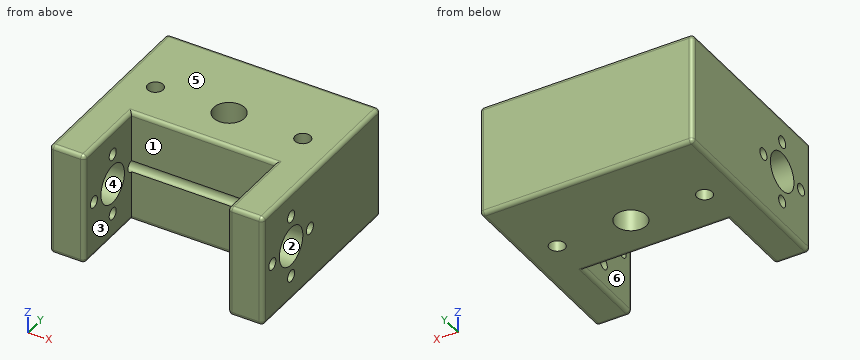
from build123d import *

# Parameters (mm, degrees)
BOSS_EXTRUDE1_DEPTH = 14.5
SKETCH2_R           = 5
SKETCH2_R_2         = 1.5
CUT_EXTRUDE1_DEPTH  = 63.130910182
SKETCH3_R           = 4
SKETCH3_R_2         = 2
CUT_EXTRUDE2_DEPTH  = 48.140746706
FILLET1_R           = 1


with BuildPart() as part:
    # Sketch1 → Boss-Extrude1 (new, symmetric)
    with BuildSketch(Plane.XY):
        Polygon((-27.5, -25), (-18.5, -25), (-18.5, -5), (18.5, -5), (18.5, -25), (27.5, -25), (27.5, 25), (-27.5, 25), align=None)
    extrude(amount=BOSS_EXTRUDE1_DEPTH, both=True)

    # Sketch2 → Cut-Extrude1 (cut, through all)
    with BuildSketch(Plane(origin=(27.5, 0, 0), x_dir=(0, 0, -1), z_dir=(1, 0, 0))):
        with Locations((0, -13)):
            Circle(SKETCH2_R)
        with Locations((0, -21)):
            Circle(SKETCH2_R_2)
        with Locations((-8, -13)):
            Circle(SKETCH2_R_2)
        with Locations((0, -5)):
            Circle(SKETCH2_R_2)
        with Locations((8, -13)):
            Circle(SKETCH2_R_2)
    extrude(amount=-CUT_EXTRUDE1_DEPTH, mode=Mode.SUBTRACT)

    # Sketch3 → Cut-Extrude2 (cut, through all)
    with BuildSketch(Plane.XY.offset(14.5)):
        with Locations((0, 6)):
            Circle(SKETCH3_R)
        with Locations((-19, 6)):
            Circle(SKETCH3_R_2)
        with Locations((19, 6)):
            Circle(SKETCH3_R_2)
    extrude(amount=-CUT_EXTRUDE2_DEPTH, mode=Mode.SUBTRACT)

    # Fillet1
    fillet1_edges = [part.edges().sort_by_distance(p)[0] for p in [
        (-18.5, -15, -14.5),
        (-23, -25, -14.5),
        (23, -25, 14.5),
        (-27.5, 0, -14.5),
        (0, 25, -14.5),
        (27.5, 0, -14.5),
        (23, -25, -14.5),
        (18.5, -15, -14.5),
        (27.5, 0, 14.5),
        (-18.5, -25, 0),
        (-27.5, -25, 0),
        (-27.5, 25, 0),
        (27.5, 25, 0),
        (27.5, -25, 0),
        (18.5, -25, 0),
        (0, 25, 14.5),
        (-27.5, 0, 14.5),
        (-23, -25, 14.5),
        (-18.5, -15, 14.5),
        (0, -5, 14.5),
        (18.5, -15, 14.5),
        (0, -5, -14.5),
    ]]
    fillet(fillet1_edges, radius=FILLET1_R)


solid = part.part
Verification items for the finished model (mm, model axes). Face numbers are marked on the shaded views. A direction names the side the tool comes from. Coordinates: 2 decimals unless noted, no trailing zeros. Order: outer loops, then holes, each group sorted by start corner. A loop starts at its lowest first (then second) coordinate and runs counter-clockwise, first axis right, second up.
Item 1: Release check for a two-part mould opening along Y. For the marked faces 1, 2, 3 and 4 record: +Y half, -Y half, draft (parallel to the pull), parting line (faces both ways), or undercut.
Filled in:
face 1: -Y half
face 2: undercut
face 3: draft
face 4: undercut
Item 2: Section check B-B, the plane x = 0. Enter the section's corners in (y, z), then the cut area to 3 significant figures.
Filled in:
outline: (-5, -13.5) arc R1 ccw to (-4, -14.5) - (2, -14.5) - (2, 14.5) - (-4, 14.5) arc R1 ccw to (-5, 13.5) - (-5, 1.5) arc R1.5 cw to (-5, -1.5) - close; (10, -14.5) - (24, -14.5) arc R1 ccw to (25, -13.5) - (25, 13.5) arc R1 ccw to (24, 14.5) - (10, 14.5) - close
area: 634 mm2
Item 3: Section check D-D, the plane y = 9. Enter the section's corners in (x, z).
Filled in:
outline: (-27.5, -13.5) arc R1 ccw to (-26.5, -14.5) - (-2.65, -14.5) - (-2.65, 14.5) - (-26.5, 14.5) arc R1 ccw to (-27.5, 13.5) - close; (2.65, -14.5) - (26.5, -14.5) arc R1 ccw to (27.5, -13.5) - (27.5, 13.5) arc R1 ccw to (26.5, 14.5) - (2.65, 14.5) - close
Item 4: Material ranges on L1, parallel to Y at x = -22.75, z = 0; L2, parallel to X at y = -10.5, z = 7.5; L3, parallel to X at y = 5, z = -10, recorded low to high.
Filled in:
L1: y = -25 to -22.5, -19.5 to -18, -8 to -6.5, -3.5 to 25
L2: x = -27.5 to -18.5, 18.5 to 27.5
L3: x = -27.5 to -20.73, -17.27 to -3.87, 3.87 to 17.27, 20.73 to 27.5
Item 5: Access from +Z, -Z, +X, -X, +Y, -Y to the whole of each face (thin tool, end or side, straight path). Record for the marked faces 5 and 6.
Filled in:
face 5: +Z, +X, -X, +Y, -Y
face 6: +Z, -Z, -Y
Item 6: Section check A-A, the plane z = -8. Enter the section's corners in (x, y), then the cut area to 3 significant figures.
Filled in:
outline: (-27.5, -24) arc R1 ccw to (-26.5, -25) - (-19.5, -25) arc R1 ccw to (-18.5, -24) - (-18.5, -14.5) - (-27.5, -14.5) - close; (-27.5, -11.5) - (-18.5, -11.5) - (-18.5, -5) - (18.5, -5) - (18.5, -11.5) - (27.5, -11.5) - (27.5, 24) arc R1 ccw to (26.5, 25) - (-26.5, 25) arc R1 ccw to (-27.5, 24) - close; (18.5, -24) arc R1 ccw to (19.5, -25) - (26.5, -25) arc R1 ccw to (27.5, -24) - (27.5, -14.5) - (18.5, -14.5) - close; hole circle Ø4 at (-19, 6); hole circle Ø8 at (0, 6); hole circle Ø4 at (19, 6)
area: 1,880 mm2
Item 7: Section check C-C, the plane y = -9. Enter the section's corners in (x, z).
Filled in:
outline: (-27.5, -13.5) arc R1 ccw to (-26.5, -14.5) - (-19.5, -14.5) arc R1 ccw to (-18.5, -13.5) - (-18.5, -3) - (-27.5, -3) - close; (-27.5, 3) - (-18.5, 3) - (-18.5, 13.5) arc R1 ccw to (-19.5, 14.5) - (-26.5, 14.5) arc R1 ccw to (-27.5, 13.5) - close; (18.5, -13.5) arc R1 ccw to (19.5, -14.5) - (26.5, -14.5) arc R1 ccw to (27.5, -13.5) - (27.5, -3) - (18.5, -3) - close; (18.5, 3) - (27.5, 3) - (27.5, 13.5) arc R1 ccw to (26.5, 14.5) - (19.5, 14.5) arc R1 ccw to (18.5, 13.5) - close
Item 8: Depth check by flat-ended pin: pin 1 (8 mm diameter, centred on y = -13, z = 0, fed in from -X); pin 2 (1 mm diameter, centred on x = 7.5, z = 1.5, fed in from -Y); pin 3 (8 mm diameter, centred on x = -8, y = -8.5, fed in from +Z). Enter the tip coordinate at first touch or a pass-through.
Filled in:
pin 1: passes through
pin 2: stops at y = -5
pin 3: stops at z = 14.37
